Answer from the drawing. Dimensions are ordinates in mm from the lowest x, y and z of the part. Round coordinates to 2 decimals unless told otherwise and drop trailing zeros. Loops run counter-clockwise (first coordinate to the right, second up) from the corner with the lowest first, then second, coordinate; pieces in that order, holes last. Notation, with made-up numbers: M 21.5,46 L 57.5,46 A18 cw 57.5,69 Z; hole C 21,-25 d6. An arc over 180 degrees is marked long. Answer as a JSON object with one key per item and string values.
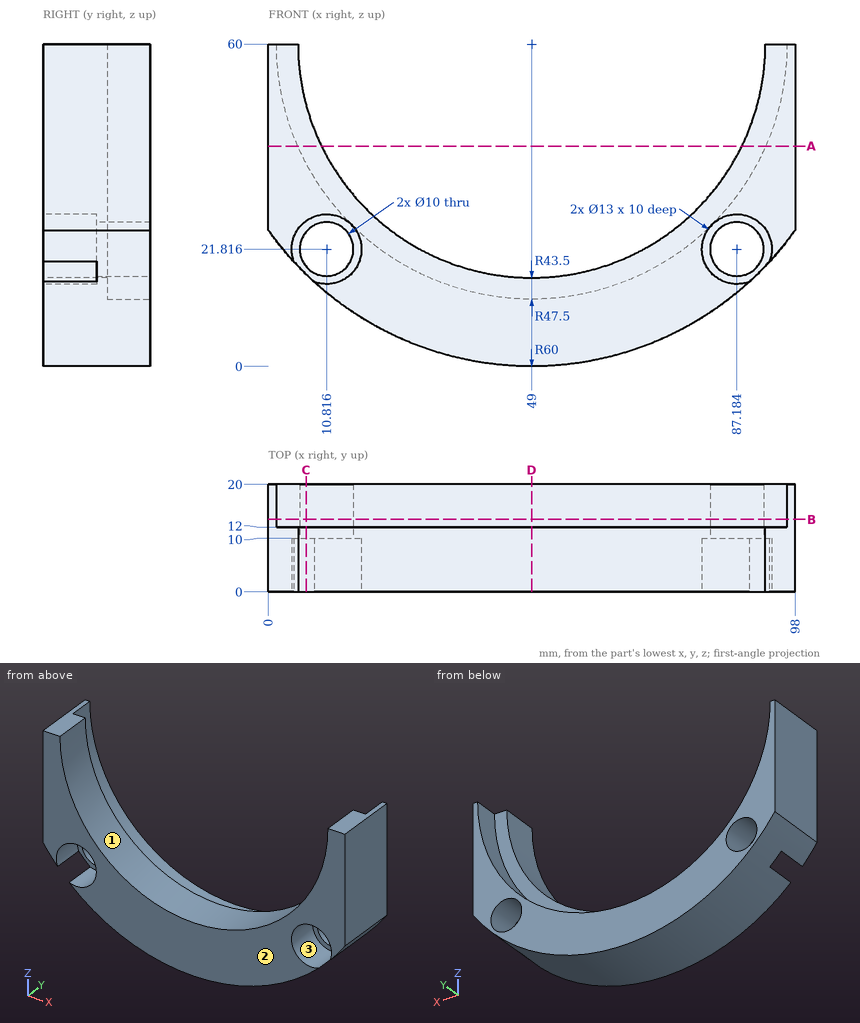
Item 1: The part is cut by section A-A (z = 41). Give the vertices of the cut face in (x, y).
Values follow:
{"outline": "M 0,0 L 9.87,0 L 9.87,12 L 5.47,12 L 5.47,20 L 0,20 Z; M 88.13,0 L 98,0 L 98,20 L 92.53,20 L 92.53,12 L 88.13,12 Z"}
Item 2: The part is cut by section D-D (x = 49). Give the vertices of the cut face in (y, z).
Values follow:
{"outline": "M 0,0 L 20,0 L 20,12.5 L 12,12.5 L 12,16.5 L 0,16.5 Z"}
Item 3: Straight lines are drawn through the part: line 1 (Y direction, x = 71, z = 21.5); line 2 (X direction, y = 8, z = 44); line 3 (Z direction, x = 48.5, y = 8.75). For each, find the intervals that lie inside material, in ascending order.
Values follow:
{"line 1": "0 to 12", "line 2": "0 to 8.55, 89.45 to 98", "line 3": "0 to 16.5"}
Item 4: Determine the mould class of the marked faces 1, 2 and 3 for opening direction Z: released by +Z, released by -Z, zero draft, split by the parting line, or undercut.
Values follow:
{"face 1": "released by +Z", "face 2": "zero draft", "face 3": "undercut"}
Item 5: The part is cut by section B-B (y = 13.5). Give the vertices of the cut face in (x, z), then the cut area to 3 significant figures.
Values follow:
{"outline": "M 0,25.37 A60 ccw 98,25.37 L 98,60 L 96.5,60 A47.5 cw 1.5,60 L 0,60 Z; hole C 10.82,21.82 d10; hole C 87.18,21.82 d10", "area": "1,440 mm^2"}
Item 6: Flat-ended cylindrical pins translate along their axes: P1, Ø12, axis at y = 14.5, z = 17.5, coming from the -X side; P2, Ø4, axis at x = 85, z = 24, coming from the -Y side; P3, Ø3, axis at y = 13.5, z = 6.5, coming from the +X side. Find the tip coordinate at first contact, or state that the pin passes through.
Values follow:
{"P1": "x = 1.38", "P2": "y = 10", "P3": "x = 78.93"}
Item 7: The part is cut by section C-C (x = 7). Give the vertices of the cut face in (y, z) (1 decimal), then the cut area to 3 significant figures.
Values follow:
{"outline": "M 0,27.1 L 10,27.1 L 10,25 L 20,25 L 20,37.8 L 12,37.8 L 12,48.7 L 0,48.7 Z; M 10,17.2 L 20,17.2 L 20,18.6 L 10,18.6 Z", "area": "380 mm^2"}
